Could you check a few things on this model? Use its own coordinates, in mm. Face numbers are marked on the shaded views. A direction names the side the tool comes from. Give positions to 0.01 mm unless a question says otherwise; leave off trailing zeros. Order: outer loops, then holes, each group sorted by start corner. A loop starts at its lowest first (then second) coordinate and runs counter-clockwise, first axis right, second up. Notation, with made-up numbers: (17.25, 89.5) -> (38.25, 89.5) arc R34 ccw to (38.25, 123.5) -> close; hole circle Ø2 at (82.5, 86.25). An arc over 180 degrees is marked (long way). Answer as CSV lines item,"result". Start each with the question number.
(1) We'd pull the mould along Y, two halves only. Please class the marked faces 1, 2 and 3: released by +Y, released by -Y, zero draft, split by the parting line, or undercut.
(2) On a 3-axis mill with a long thin cutter (end or side, diameter ignored), from which of +Z, -Z, +X, -X, +Y, -Y can I reach the whole of each face in a straight line? I mean the marked faces 4 and 5. Say none if no direction works.
(3) I want a section at A-A (y = 7). Please give me the cut outline in (x, z).
(4) I need wall thicknesses on L1, parallel to Y at x = -1, z = -1; L2, parallel to Z at x = 0, y = 0.2; L3, parallel to Z at x = 0, y = 8.5. Which ranges of each line are inside material? Lowest first, please.
(5) I want a section at B-B (y = 1.75). Please give me the cut outline in (x, z), plus the area to 3 significant figures.
(6) Will these pins go through, and if not, where does the flat tip stop? pin 1 Ø1.5 at (y, z) = (1.5, 4) entering from +X; pin 2 Ø1.5 at (x, y) = (-3.5, 7.5) entering from -Z; pin 3 Ø3 at (x, z) = (-2, -0.5) entering from -Y.
```python
from build123d import *

# Parameters (mm, degrees)
SKETCH2_R           = 5.4
CUT_EXTRUDE1_DEPTH  = 0.5
SKETCH4_R           = 0.3
BOSS_EXTRUDE2_DEPTH = 5
SKETCH5_R           = 1.27
SKETCH5_R_2         = 1.1
CUT_EXTRUDE2_DEPTH  = 0.01
CUT_EXTRUDE3_DEPTH  = 0.01
SKETCH7_R           = 1.25
CUT_EXTRUDE4_DEPTH  = 3
SKETCH8_R           = 4.5
CUT_EXTRUDE5_DEPTH  = 2
SKETCH12_R          = 1.25
BOSS_EXTRUDE4_DEPTH = 0.5
BOSS_EXTRUDE4_TAPER = 45
FILLET3_R           = 1
SKETCH13_W          = 1
SKETCH13_H          = 0.5


with BuildPart() as part:
    # Sketch1 → Revolve1 (revolve)
    with BuildSketch(Plane.XY):
        Polygon((0, 0), (0, 9), (5.8, 9), (6, 0), align=None)
    revolve(axis=Axis((0, 0, 0), (0, 1, 0)))

    # Sketch2 → Cut-Extrude1 (cut)
    with BuildSketch(Plane.XZ):
        Circle(SKETCH2_R)
    extrude(amount=-CUT_EXTRUDE1_DEPTH, mode=Mode.SUBTRACT)

    # Sketch4 → Boss-Extrude2 (add)
    with BuildSketch(Plane.XZ.offset(-0.5)):
        with Locations((0, -3.81)):
            Circle(SKETCH4_R)
        with Locations((0, 3.81)):
            Circle(SKETCH4_R)
    extrude(amount=BOSS_EXTRUDE2_DEPTH)

    # Sketch5 → Cut-Extrude2 (cut)
    with BuildSketch(Plane(origin=(0, 9, 0), x_dir=(1, 0, 0), z_dir=(0, 1, 0))):
        with Locations((0, -3.8)):
            Circle(SKETCH5_R)
        with Locations((0, -3.8)):
            Circle(SKETCH5_R_2, mode=Mode.SUBTRACT)
    extrude(amount=-CUT_EXTRUDE2_DEPTH, mode=Mode.SUBTRACT)

    # Sketch6 → Cut-Extrude3 (cut)
    with BuildSketch(Plane(origin=(0, 9, 0), x_dir=(1, 0, 0), z_dir=(0, 1, 0))):
        Polygon((-0.175, -3.05), (0.175, -3.05), (0.175, -3.625), (0.75, -3.625), (0.75, -3.975), (0.175, -3.975), (0.175, -4.55), (-0.175, -4.55), (-0.175, -3.975), (-0.75, -3.975), (-0.75, -3.625), (-0.175, -3.625), align=None)
    extrude(amount=-CUT_EXTRUDE3_DEPTH, mode=Mode.SUBTRACT)

    # Sketch7 → Cut-Extrude4 (cut)
    with BuildSketch(Plane(origin=(0, 9, 0), x_dir=(1, 0, 0), z_dir=(0, 1, 0))):
        Circle(SKETCH7_R)
    extrude(amount=-CUT_EXTRUDE4_DEPTH, mode=Mode.SUBTRACT)

    # Sketch8 → Cut-Extrude5 (cut)
    with BuildSketch(Plane(origin=(0, 6, 0), x_dir=(1, 0, 0), z_dir=(0, 1, 0))):
        Circle(SKETCH8_R)
    extrude(amount=CUT_EXTRUDE5_DEPTH, mode=Mode.SUBTRACT)

    # Sketch12 → Boss-Extrude4 (add)
    with BuildSketch(Plane.XZ.offset(-0.5)):
        with Locations((0, 3.81)):
            Circle(SKETCH12_R)
        with Locations((0, -3.81)):
            Circle(SKETCH12_R)
    extrude(amount=BOSS_EXTRUDE4_DEPTH, taper=BOSS_EXTRUDE4_TAPER)

    # Fillet3
    fillet3_edges = [part.edges().sort_by_distance(p)[0] for p in [
        (-0.75, 0, 3.81),
        (-0.75, 0, -3.81),
    ]]
    fillet(fillet3_edges, radius=FILLET3_R)

    # Sketch13 → Cut-Revolve1 (revolve, cut)
    with BuildSketch(Plane.XY):
        with Locations((6.1, 2.75)):
            Rectangle(SKETCH13_W, SKETCH13_H)
    revolve(axis=Axis((0, 0, 0), (0, 1, 0)), mode=Mode.SUBTRACT)


solid = part.part
```
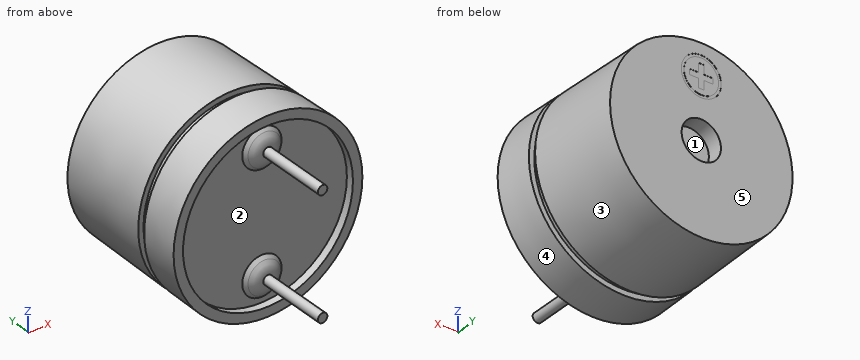
Final values:
1,face 1,"undercut"
1,face 2,"released by -Y"
1,face 3,"released by +Y"
2,face 4,"+Y"
2,face 5,"+Z, -Z, +X, -X, +Y"
3,outline,"circle Ø11.69 at (0, 0); hole circle Ø9 at (0, 0)"
4,L1,"0.5 to 6, 8 to 9"
4,L2,"-6 to -5.4, -4.75 to -2.87, 2.87 to 4.75, 5.4 to 6"
4,L3,"-5.81 to -1.25, 1.25 to 5.81"
5,outline,"circle Ø11.92 at (0, 0)"
5,area,"112 mm²"
6,pin 1,"x = 5"
6,pin 2,"z = -5.14"
6,pin 3,"y = 0.5"
